For this review, take the finished solid that the model builds, in its own axes (mm). Give positions to 0.01 mm unless a question says otherwise; leave off trailing zeros. Loops run counter-clockwise (first coordinate to the right, second up) from the corner with the lowest first, then second, coordinate; pieces in that order, holes last. Notation, with made-up numbers: (20.25, -5) -> (59.25, -5) arc R8 ccw to (59.25, 0) -> close; hole circle Ø5 at (66, 24). An arc over 180 degrees is marked (long way). Write each question's results on one line, items separated by ' | '. Start each with the question number.
```python
from build123d import *

# Parameters (mm, degrees)
BOSS_EXTRUDE1_DEPTH = 24
BOSS_EXTRUDE2_DEPTH = 48
SKETCH3_R           = 3
BOSS_EXTRUDE3_DEPTH = 16.34


with BuildPart() as part:
    # Sketch1 → Boss-Extrude1 (new, symmetric)
    with BuildSketch(Plane.XY):
        with BuildLine():
            Line((0, 0), (6.458695376, 6.458695376))
            ThreePointArc((6.458695376, 6.458695376), (6.941658289, 6.588104899), (7.29521168, 6.234551508))
            Line((7.29521168, 6.234551508), (9.659258263, -2.588190451))
            ThreePointArc((9.659258263, -2.588190451), (9.305704872, -3.200562887), (8.693332437, -2.847009496))
            Line((8.693332437, -2.847009496), (6.77757359, 4.302699856))
            ThreePointArc((6.77757359, 4.302699856), (6.424020199, 4.656253246), (5.941057286, 4.526843724))
            Line((5.941057286, 4.526843724), (0.707106781, -0.707106781))
            ThreePointArc((0.707106781, -0.707106781), (0, -0.707106781), (0, 0))
        make_face()
    extrude(amount=BOSS_EXTRUDE1_DEPTH, both=True)

    # Sketch2 → Boss-Extrude2 (add)
    with BuildSketch(Plane.XY.offset(24)):
        with BuildLine():
            Line((0.707106781, -0.707106781), (5.941057286, 4.526843724))
            ThreePointArc((5.941057286, 4.526843724), (6.424020199, 4.656253246), (6.77757359, 4.302699856))
            Line((6.77757359, 4.302699856), (8.693332437, -2.847009496))
            Line((8.693332437, -2.847009496), (0.707106781, -0.707106781))
        make_face()
    extrude(amount=-BOSS_EXTRUDE2_DEPTH)

    # Sketch3 → Boss-Extrude3 (add)
    with BuildSketch(Plane(origin=(-0.129409523, -0.482962913, 0), x_dir=(0.9659258262890683, -0.25881904510252096, 0), z_dir=(-0.25881904510252096, -0.9659258262890683, 0))):
        with Locations((5, 0)):
            Circle(SKETCH3_R)
    extrude(amount=BOSS_EXTRUDE3_DEPTH)


solid = part.part
```
1. We need section A-A (z = -16). Write out the cut boundary in (x, y), plus the area to 3 significant figures.
2. Wall thickness on L1, parallel to Z at x = 2.25, y = -11.75; L2, parallel to X at y = -9.75, z = -1.5; L3, parallel to Y at x = 3, z = 16: over which ranges is each line inside the solid? List them lowest first.
3. For pin 1 Ø1.5 at (x, z) = (-0.5, -5.5) entering from -Y; pin 2 Ø4 at (x, z) = (-1, 19) entering from -Y; pin 3 Ø4 at (x, z) = (3.5, 0.5) entering from +Y; pin 4 Ø4 at (x, y) = (7.5, -15.5) entering from +Z, all flat-tipped, find the tip position at first contact; note any pin that passes through.
4. We need section B-B (y = 3.75). Write out the cut boundary in (x, z).
Response:
1) outline: (0, 0) arc R0.5 ccw to (0.71, -0.71) -> (8.69, -2.85) arc R0.5 ccw to (9.66, -2.59) -> (7.3, 6.23) arc R0.5 ccw to (6.46, 6.46) -> close | area: 48.5 mm2
2) L1: z = -2.99 to 2.99 | L2: x = -0.13 to 5.25 | L3: y = -1.32 to 3
3) pin 1: stops at y = -0.84 | pin 2: stops at y = -0.85 | pin 3: stops at y = 5.5 | pin 4: passes through
4) outline: (3.75, -24) -> (7.96, -24) -> (7.96, 24) -> (3.75, 24) -> close
